from build123d import *

# Parameters (mm, degrees)
F0_R     = 11
F1_DEPTH = 5


with BuildPart() as f1:
    # F0 (on Front) → F1 (new body)
    with BuildSketch(Plane.XZ):
        with BuildLine():
            ThreePointArc((13.228757, -10), (12.344873, -9.467707), (12.401959, -8.4375))
            ThreePointArc((12.401959, -8.4375), (0, 15), (-12.401959, -8.4375))
            ThreePointArc((-12.401959, -8.4375), (-12.344873, -9.467707), (-13.228757, -10))
            Line((-13.228757, -10), (-18.228757, -10))
            Line((-18.228757, -10), (-18.228757, -15))
            Line((-18.228757, -15), (18.228757, -15))
            Line((18.228757, -15), (18.228757, -10))
            Line((18.228757, -10), (13.228757, -10))
        make_face()
        Circle(F0_R, mode=Mode.SUBTRACT)
    extrude(amount=F1_DEPTH)


solid = f1.part
The model under review builds one solid part; all positions refer to its coordinate system, in mm. A direction names the side the tool comes from. Coordinates: 2 decimals unless noted, no trailing zeros. Write each loop counter-clockwise with the first axis right and the second up, starting at its lowest first coordinate (ties: lowest second). Pieces come first, ordered by that corner, then holes. Notation, with made-up numbers: M 51,17.5 L 70,17.5 A33 ccw 70,45.5 Z; hole C 58,55.5 d1. An arc over 180 degrees is marked long. Put each result on its own line as item: value.
1) Add section A-A on x = 0. Give the boundary of the cut face in (y, z).
Computed:
outline: M -5,-15 L 0,-15 L 0,-11 L -5,-11 Z; M -5,11 L 0,11 L 0,15 L -5,15 Z
2) Add section B-B on z = 0. Give the boundary of the cut face in (x, y), then the cut area to 3 significant figures.
Computed:
outline: M -15,-5 L -11,-5 L -11,0 L -15,0 Z; M 11,-5 L 15,-5 L 15,0 L 11,0 Z
area: 40.0 mm2
3) Add section D-D on x = -16. Give the boundary of the cut face in (y, z), then the cut area to 3 significant figures.
Computed:
outline: M -5,-15 L 0,-15 L 0,-10 L -5,-10 Z
area: 25.0 mm2
4) For faces 1 (the flat face through (16, -2, -10)), 2 (the flat face through (0, -2, -15)), list the 3-axis set-ups (+Z, -Z, +X, -X, +Y, -Y) from which the entire face can be reached by the end or side of a thin tool; tool diameter is ignored.
Computed:
face 1: +X, +Y, -Y
face 2: -Z, +X, -X, +Y, -Y
5) Add section C-C on y = -3.1. Give the boundary of the cut face in (x, z), then the cut area to 3 significant figures.
Computed:
outline: M -18.23,-15 L 18.23,-15 L 18.23,-10 L 13.23,-10 A1 cw 12.4,-8.44 A15 ccw long -12.4,-8.44 A1 cw -13.23,-10 L -18.23,-10 Z; hole C 0,0 d22
area: 433 mm2
6) Wall thickness on probe 1 along Z at (x, y) = (0, -2.4); probe 2 along X at (y, z) = (-2.15, -7.5); probe 3 along X at (y, z) = (-3.3, 5.75): over which ranges is each line inside the solid? List them lowest first. Write a range as [from, to].
Computed:
probe 1: z = [-15, -11], [11, 15]
probe 2: x = [-12.99, -8.05], [8.05, 12.99]
probe 3: x = [-13.85, -9.38], [9.38, 13.85]
7) Clearance check with flat-ended pins moving along their axes: pin 1 Ø17.5 at (x, z) = (0, 0) entering from -Y; pin 2 Ø2 at (y, z) = (-1, -8) entering from -X. State where each tip first meets the part, or that it passes through.
Computed:
pin 1: passes through
pin 2: stops at x = -13.27
8) Draft analysis for pull direction X (two halves, no side actions). For faces 3 (the flat face through (-16, -2, -10)), 4 (the cylindrical face through (12.35, -2.46, -9.48)), 5 (the cylindrical face through (-2.38, -2.46, -10.74)), state which applies: released by +X, released by -X, zero draft, split by the parting line, or undercut.
Computed:
face 3: zero draft
face 4: released by +X
face 5: undercut
